Autodesk Inventor part; units mm, degrees
ref_plane "YZ Plane" through (0, 0, 0) normal (1, 0, 0) x (0, 1, 0)
ref_plane "XZ Plane" through (0, 0, 0) normal (0, 1, 0) x (-1, 0, 0)
ref_plane "XY Plane" through (0, 0, 0) normal (0, 0, 1) x (1, 0, 0)
sketch "Sketch1" plane through (0, 0, 0) normal (1, 0, 0) x (0, 1, 0)
  line L0 (0, 0) -> (4.7625, 0)
  line L1 (4.7625, 0) -> (4.7625, -168.8592)
  line L2 (4.7625, -168.8592) -> (0, -168.8592)
  line L3 (0, -168.8592) -> (0, 0)
  dimension "d1" = 4.7625
  dimension "d2" = 168.8592
extrude "Extrusion1" add sketch "Sketch1" along normal blind 0.7937
sketch "Sketch2" plane through (0, 0, -168.8592) normal (0, 0, -1) x (-1, 0, 0)
  line L0 (-0.7937, 0) -> (-0.7937, 4.7625)
  line L1 (-0.7937, 0) -> (91.9162, 0)
  line L2 (91.9162, 0) -> (91.9162, 4.7625)
  line L3 (91.9162, 4.7625) -> (-0.7937, 4.7625)
  line L4 (-0.7937, 4.7625) -> (-0.7937, 0)
  point P0 (0, 0)
  dimension "d5" = 92.71
  dimension "d6" = 4.7625
extrude "Extrusion2" add sketch "Sketch2" against normal blind 0.7937
sketch "Sketch3" plane through (-91.9162, 0, -168.8592) normal (-1, 0, 0) x (0, 0, 1)
  line L0 (168.8592, 4.7625) -> (168.8592, 0)
  line L1 (0, 0) -> (168.8592, 0)
  line L2 (168.8592, 0) -> (168.8592, 4.7625)
  line L3 (168.8592, 4.7625) -> (0, 4.7625)
  line L4 (0, 4.7625) -> (0, 0)
extrude "Extrusion3" add sketch "Sketch3" against normal blind 0.7937
sketch "Sketch4" plane through (-91.9162, 0, 0) normal (0, 0, 1) x (1, 0, 0)
  line L0 (0, 0) -> (0, 4.7625)
  line L1 (91.9162, 4.7625) -> (92.71, 4.7625)
  line L2 (0, 0) -> (92.71, 0)
  line L3 (92.71, 0) -> (92.71, 4.7625)
  line L4 (92.71, 4.7625) -> (0, 4.7625)
  line L5 (0, 4.7625) -> (0, 0)
  point P0 (91.9162, 0)
extrude "Extrusion4" add sketch "Sketch4" against normal blind 0.7937
sketch "Sketch7" plane through (-36.0362, 0, 0) normal (0, 0, 1) x (1, 0, 0)
  circle A0 centre (-9.525, 2.3812) radius 2.2098
  point P0 (-55.88, 0)
  point P1 (36.83, 0)
extrude "Extrusion5" cut sketch "Sketch7" against normal blind 0.7937
sketch "Sketch6" plane through (0.7937, 0, -168.8592) normal (0, 0, -1) x (-1, 0, 0)
  circle A0 centre (46.355, 2.3813) radius 2.2098
  point P0 (0, 0)
  point P1 (92.71, 0)
extrude "Extrusion6" cut sketch "Sketch6" against normal blind 0.7937
properties part number "Back rubber bands"
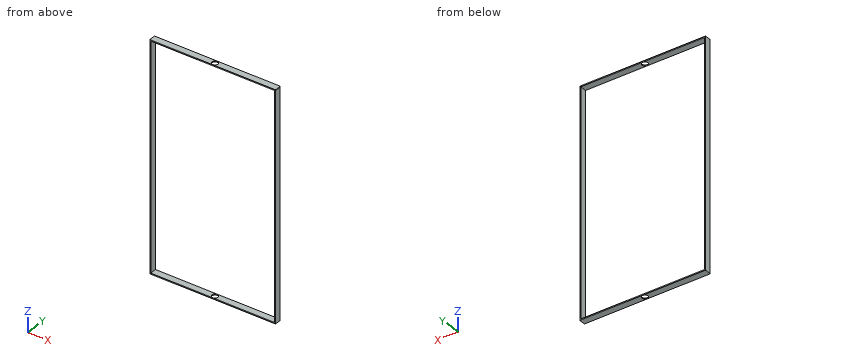
Source: CAD feature listing. Evaluate the final solid. Frame: model axes, mm. Coordinates: 2 decimals unless noted, no trailing zeros. Order: outer loops, then holes, each group sorted by start corner. A loop starts at its lowest first (then second) coordinate and runs counter-clockwise, first axis right, second up.
Item 1: First-contact query: P1, Ø12, axis at x = -8.5, z = -25.5, coming from the +Y side. Flat tip, straight axial feed; report the tip coordinate or a pass-through.
Output values:
P1: passes through
Item 2: Cut plane A-A (x = -82.5). Return loops of the section in (y, z), plus the area to 3 significant figures.
Output values:
outline: (0, -168.86) - (4.76, -168.86) - (4.76, -168.07) - (0, -168.07) - close; (0, -0.79) - (4.76, -0.79) - (4.76, 0) - (0, 0) - close
area: 7.56 mm2
Item 3: Cut plane B-B (z = -34.5). Return loops of the section in (x, y), plus the area to 3 significant figures.
Output values:
outline: (-91.92, 0) - (-91.12, 0) - (-91.12, 4.76) - (-91.92, 4.76) - close; (0, 0) - (0.79, 0) - (0.79, 4.76) - (0, 4.76) - close
area: 7.56 mm2
Item 4: Material intervals for line 1 (Z direction, x = -52, y = 1.35); line 2 (X direction, y = 1.2, z = -50.5), sorted ascending.
Output values:
line 1: z = -168.86 to -168.07, -0.79 to 0
line 2: x = -91.92 to -91.12, 0 to 0.79
